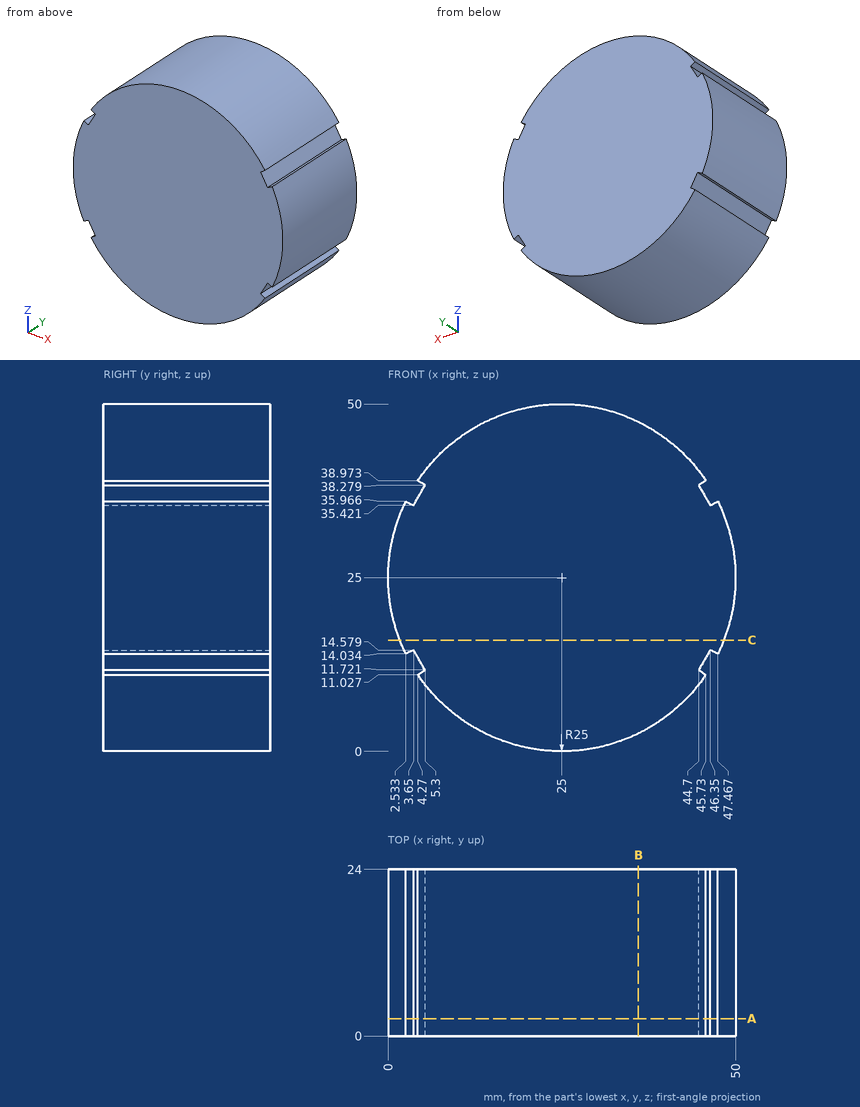
Study the drawing (mm; zero at the part's minimum x, y, z) and answer. Give positions to 0.01 mm unless a question says otherwise; leave off trailing zeros. Loops run counter-clockwise (first coordinate to the right, second up) from the corner with the lowest first, then second, coordinate; pieces in that order, holes last. Notation, with made-up numbers: (65.25, 52.25) - (72.25, 52.25) arc R25 ccw to (72.25, 91.25) - close; hole circle Ø11 at (7.5, -26). An arc over 180 degrees is marked (long way). Answer in a Markdown table with one row per item. Add a question column.
Q1. Consider line 1 along X through (y, z) = (3, 27.5) (1 decimal); line 2 along X through (y, z) = (15.5, 25.5) (1 decimal); line 3 along Z through (x, y) = (44.5, 3) (1 decimal). Determine where each line is inside the solid, lowest interval first.
Q2. The part is cut by section A-A (y = 2.5). Determine the outline of the cut face in (x, z).
Q3. The part is cut by section B-B (x = 36). Determine the outline of the cut face in (y, z), and give its area (3 significant figures).
Q4. Each of these flat-tipped pins is pushed along its axis until it touches: P1, Ø10, axis at y = 2.5, z = 27, coming from the +X side; P2, Ø3, axis at y = 6.5, z = 42.5, coming from the +X side; P3, Ø12, axis at y = 15.5, z = 34, coming from the -X side. Where does it stop, or does it pass through?
Q5. The part is cut by section C-C (z = 16). Determine the outline of the cut face in (x, y).
Solution:
| question | item | result |
|---|---|---|
| 1 | line 1 | x = 0.1 to 49.9 |
| 1 | line 2 | x = 0 to 50 |
| 1 | line 3 | z = 9.4 to 40.6 |
| 2 | outline | (2.53, 14.03) - (3.65, 14.58) - (5.3, 11.72) - (4.27, 11.03) arc R25 ccw to (45.73, 11.03) - (44.7, 11.72) - (46.35, 14.58) - (47.47, 14.03) arc R25 ccw to (47.47, 35.97) - (46.35, 35.42) - (44.7, 38.28) - (45.73, 38.97) arc R25 ccw to (4.27, 38.97) - (5.3, 38.28) - (3.65, 35.42) - (2.53, 35.97) arc R25 ccw to start |
| 3 | outline | (0, 2.55) - (24, 2.55) - (24, 47.45) - (0, 47.45) - close |
| 3 | area | 1,080 mm² |
| 4 | P1 | stops at x = 50 |
| 4 | P2 | stops at x = 44.21 |
| 4 | P3 | stops at x = 0.18 |
| 5 | outline | (1.68, 0) - (48.32, 0) - (48.32, 24) - (1.68, 24) - close |
